Geometry: final body of the model. Coordinates: model frame, mm. A direction names the side the tool comes from. Give positions to 0.01 mm unless a question says otherwise; leave off trailing zeros. Write each loop counter-clockwise with the first axis right and the second up, starting at its lowest first coordinate (ties: lowest second). Pieces come first, ordered by that corner, then holes.
```python
from build123d import *

# Parameters (mm, degrees)
ESBO_O1_W                = 17.000001856
ESBO_O1_H                = 13.999999967
RESSALTO_EXTRUS_O1_DEPTH = 12.000000396
ESBO_O2_W                = 12.500001117
ESBO_O2_H                = 10.30000049
CORTE_EXTRUS_O1_DEPTH    = 14.999999966
ESBO_O3_W                = 7.999999915
ESBO_O3_H                = 3.000000085
RESSALTO_EXTRUS_O2_DEPTH = 6.999999285
ESBO_O4_R                = 1.75
CORTE_EXTRUS_O2_DEPTH    = 13.000000396
ESBO_O5_W                = 7.999999915
ESBO_O5_H                = 3.000000085
RESSALTO_EXTRUS_O3_DEPTH = 6.999999285
ESBO_O6_R                = 1.75
CORTE_EXTRUS_O3_DEPTH    = 13.000000396


with BuildPart() as part:
    # Esboço1 → Ressalto-extrusão1 (new body)
    with BuildSketch(Plane.XZ.offset(-5e-05)):
        with Locations((15.500025358, 7.000024663)):
            Rectangle(ESBO_O1_W, ESBO_O1_H)
    extrude(amount=-RESSALTO_EXTRUS_O1_DEPTH)

    # Esboço2 → Corte-extrusão1 (cut, through all)
    with BuildSketch(Plane.XY.offset(14.000024647)):
        with Locations((15.500024893, 5.150050245)):
            Rectangle(ESBO_O2_W, ESBO_O2_H)
    extrude(amount=-CORTE_EXTRUS_O1_DEPTH, mode=Mode.SUBTRACT)

    # Esboço3 → Ressalto-extrusão2 (add)
    with BuildSketch(Plane.ZY.offset(-7.00002443)):
        with Locations((10.00002469, 1.500050043)):
            Rectangle(ESBO_O3_W, ESBO_O3_H)
    extrude(amount=RESSALTO_EXTRUS_O2_DEPTH)

    # Esboço4 → Corte-extrusão2 (cut, through all)
    with BuildSketch(Plane.XZ.offset(-5e-05)):
        with Locations((3.250025213, 10.000025168)):
            Circle(ESBO_O4_R)
    extrude(amount=-CORTE_EXTRUS_O2_DEPTH, mode=Mode.SUBTRACT)

    # Esboço5 → Ressalto-extrusão3 (add)
    with BuildSketch(Plane(origin=(24.000026286, 0, 0), x_dir=(0, 0, -1), z_dir=(1, 0, 0))):
        with Locations((-10.00002469, 1.500050043)):
            Rectangle(ESBO_O5_W, ESBO_O5_H)
    extrude(amount=RESSALTO_EXTRUS_O3_DEPTH)

    # Esboço6 → Corte-extrusão3 (cut, through all)
    with BuildSketch(Plane.XZ.offset(-5e-05)):
        with Locations((27.751375675, 10.000025168)):
            Circle(ESBO_O6_R)
    extrude(amount=-CORTE_EXTRUS_O3_DEPTH, mode=Mode.SUBTRACT)


solid = part.part
```
Item 1: Reachability of faces 5 (the face through (5, 3, 9)), 6 (the face through (21.75, 5, 7)), 7 (the face through (4, 1, 6)) from +Z, -Z, +X, -X, +Y, -Y: full face, straight path, thin tool, end or side. Return the list, or none.
Found:
face 5: +Z, -Z, -X, +Y
face 6: +Z, -Z, -Y
face 7: -Z, -X, +Y, -Y
Item 2: Pull-direction query (Z, two-part tool) for faces 1 (the face through (25, 0, 9)), 2 (the face through (4.919, 1.479, 10.526)), 3 (the face through (27, 1, 6)), 4 (the face through (15, 11, 14)); classes: +Z half, -Z half, draft (parallel to the pull), parting line (faces both ways), or undercut.
Found:
face 1: draft
face 2: undercut
face 3: -Z half
face 4: +Z half
Item 3: Section C-C, the plane y = 7.5. Return the cut outline in (x, z).
Found:
outline: (7, 0) - (9.25, 0) - (9.25, 14) - (7, 14) - close; (21.75, 0) - (24, 0) - (24, 14) - (21.75, 14) - close
Item 4: Section B-B, the plane z = 3.5. Return the cut outline in (x, y).
Found:
outline: (7, 0) - (9.25, 0) - (9.25, 10.3) - (21.75, 10.3) - (21.75, 0) - (24, 0) - (24, 12) - (7, 12) - close
Item 5: Section D-D, the plane x = 26.5. Return the cut outline in (y, z), plus the area to 3 significant figures.
Found:
outline: (0, 6) - (3, 6) - (3, 8.78) - (0, 8.78) - close; (0, 11.22) - (3, 11.22) - (3, 14) - (0, 14) - close
area: 16.7 mm2
Item 6: Pin query (flat end, axial travel): pin 1 Ø3 at (x, z) = (3.25, 10) entering from +Y; pin 2 Ø6 at (y, z) = (8, 8) entering from -X; pin 3 Ø2 at (x, y) = (15, 9.5) entering from +Z; pin 4 Ø4 at (x, z) = (14, 8.5) entering from -Y. Return the tip coordinate at first contact, or that it passes through.
Found:
pin 1: passes through
pin 2: stops at x = 7
pin 3: stops at z = 14
pin 4: stops at y = 10.3
Item 7: Line query: L1, parallel to X at y = 2, z = 10; L2, parallel to X at y = 8.25, z = 7; L3, parallel to Y at x = 20.5, z = 13.5. Output: solid intervals per line, ascending.
Found:
L1: x = 0 to 1.5, 5 to 9.25, 21.75 to 26, 29.5 to 31
L2: x = 7 to 9.25, 21.75 to 24
L3: y = 10.3 to 12
Item 8: Section A-A, the plane y = 2. Return the cut outline in (x, z), plus the area to 3 significant figures.
Found:
outline: (0, 6) - (7, 6) - (7, 0) - (9.25, 0) - (9.25, 14) - (0, 14) - close; (21.75, 0) - (24, 0) - (24, 6) - (31, 6) - (31, 14) - (21.75, 14) - close; hole circle Ø3.5 at (3.25, 10); hole circle Ø3.5 at (27.75, 10)
area: 156 mm2
